For this review, take the finished solid that the model builds, in its own axes (mm). Face numbers are marked on the shaded views. A direction names the side the tool comes from. Coordinates: 2 decimals unless noted, no trailing zeros. Loops run counter-clockwise (first coordinate to the right, second up) from the corner with the lowest first, then second, coordinate; pieces in that order, holes last. Notation, with made-up numbers: M 17.25,21 L 45.25,21 A10 cw 45.25,34 Z; hole C 52.25,-28.5 d10. An arc over 180 degrees is marked long. Use one line per item in the form item = value.
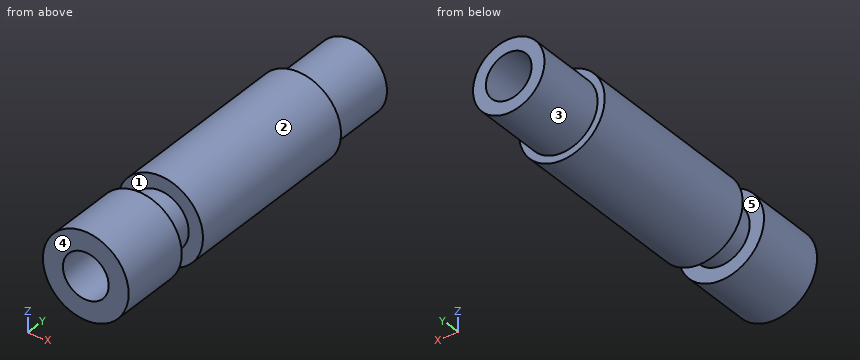
```python
from build123d import *

# Parameters (mm, degrees)
SKETCH2_R          = 1.6
CUT_EXTRUDE1_DEPTH = 26


with BuildPart() as part:
    # Sketch1 → Revolve1 (revolve)
    with BuildSketch(Plane.XY):
        Polygon((0, 0), (0, 25), (2.5, 25), (2.5, 20), (3, 20), (3, 7), (2, 7), (2, 5), (3, 5), (3, 0), align=None)
    revolve(axis=Axis((0, 0, 0), (0, 1, 0)))

    # Sketch2 → Cut-Extrude1 (cut, through all)
    with BuildSketch(Plane(origin=(0, 25, 0), x_dir=(1, 0, 0), z_dir=(0, 1, 0))):
        Circle(SKETCH2_R)
    extrude(amount=-CUT_EXTRUDE1_DEPTH, mode=Mode.SUBTRACT)


solid = part.part
```
1. Consider section D-D on y = 21.5. Write out the cut boundary in (x, z), plus the area to 3 significant figures.
Computed values:
outline = C 0,0 d5; hole C 0,0 d3.2
area = 11.6 mm2
2. Consider section C-C on y = 18.25. Write out the cut boundary in (x, z), plus the area to 3 significant figures.
Computed values:
outline = C 0,0 d6; hole C 0,0 d3.2
area = 20.2 mm2
3. Wall thickness on line 1 along Z through (x, y) = (0, 7.75); line 2 along Y through (x, z) = (1.85, 2.3); line 3 along Z through (x, y) = (0, 5.5): over which ranges is each line inside the solid? List them lowest first. Write a range as from..to.
Computed values:
line_1 = -3..-1.6, 1.6..3
line_2 = 0..5, 7..20
line_3 = -2..-1.6, 1.6..2
4. Draft analysis for pull direction Y (two halves, no side actions). For the marked faces 3, 4 and 5, state which applies: +Y half, -Y half, draft (parallel to the pull), parting line (faces both ways), or undercut.
Computed values:
face_3 = draft
face_4 = -Y half
face_5 = undercut
5. For pin 1 Ø2.5 at (x, z) = (0, 0) entering from +Y, flat-tipped, find the tip position at first contact; note if it passes through.
Computed values:
pin_1 = through
6. Tool access review of the marked faces 1 and 2: name each direction out of +Z, -Z, +X, -X, +Y, -Y from which nothing blocks a thin tool from reaching the whole face with its end or side.
Computed values:
face_1 = none
face_2 = +Y, -Y
7. Consider section A-A on x = 0. Write out the cut boundary in (y, z), plus the area to 3 significant figures.
Computed values:
outline = M 0,-3 L 5,-3 L 5,-2 L 7,-2 L 7,-3 L 20,-3 L 20,-2.5 L 25,-2.5 L 25,-1.6 L 0,-1.6 Z; M 0,1.6 L 25,1.6 L 25,2.5 L 20,2.5 L 20,3 L 7,3 L 7,2 L 5,2 L 5,3 L 0,3 Z
area = 61.0 mm2
8. Consider section B-B on z = 0. Write out the cut boundary in (x, y).
Computed values:
outline = M -3,0 L -1.6,0 L -1.6,25 L -2.5,25 L -2.5,20 L -3,20 L -3,7 L -2,7 L -2,5 L -3,5 Z; M 1.6,0 L 3,0 L 3,5 L 2,5 L 2,7 L 3,7 L 3,20 L 2.5,20 L 2.5,25 L 1.6,25 Z
